Source: CAD feature listing. Evaluate the final solid. Frame: model axes, mm. A direction names the side the tool comes from. Give positions to 0.01 mm unless a question says otherwise; leave off trailing zeros. Order: outer loops, then holes, each group sorted by start corner. A loop starts at its lowest first (then second) coordinate and runs counter-clockwise, first axis right, second up. Notation, with made-up numbers: (-33, -34) - (20, -34) arc R10 cw to (20, -27) - close; hole circle Ø8 at (-37.5, 57.25). An arc over 180 degrees is marked (long way). Write each question's results on one line, items separated by ' | '. Start each with the question number.
Item 1: Line query: line 1 along Y through (x, z) = (242, 18.25); line 2 along X through (y, z) = (0, 18); line 3 along Z through (x, y) = (-39, -187.5). Output: solid intervals per line, ascending.
Item 2: Section B-B on x = -57. Output: boundary loops of the cut face in (y, z), and give its area (3 significant figures).
Item 3: Mould query, pull axis Y, two halves, no side actions, for faces 4 (the cylindrical face through (-57.08, -126.19, 31.67)), 5 (the flat face through (0.88, 133.23, 37.99)), 6 (the flat face through (4, -26, 18.5)), 7 (the cylindrical face through (57.08, 126.19, 31.67)). Classes: released by +Y, released by -Y, zero draft, split by the parting line, or undercut.
Item 4: Section A-A on z = 42.5. Output: boundary loops of the cut face in (x, y).
Item 5: Set-up query: faces 1 (the cylindrical face through (-28.53, -205.21, 57.52)), 2 (the flat face through (1, 180, 57.031)), 3 (the flat face through (1, -179, 57.031)). Return all of +Z, -Z, +X, -X, +Y, -Y with unobstructed straight access to the full face (end or side cutting, diameter ignored); none if empty.
Item 6: Contact query for flat-ended pins moving along their axis: pin 1 Ø3 at (x, y) = (13.5, -41.5) entering from +Z; pin 2 Ø0.5 at (y, z) = (-206.5, 57.5) entering from -X; pin 3 Ø1.1 at (y, z) = (198.5, 57.5) entering from -X. Output: stop coordinate, or through.
Item 7: Section C-C on y = 53.5. Output: boundary loops of the cut face in (x, z), and give its area (3 significant figures).
Item 8: Section D-D on x = 123. Output: boundary loops of the cut face in (y, z).
```python
from build123d import *

# Parameters (mm, degrees)
SALIENTE_EXTRUIR1_DEPTH     = 271
CORTAR_EXTRUIR9_DEPTH       = 372.904084134
CORTAR_EXTRUIR9_DEPTH_BACK  = 372.904084134
CROQUIS4_R                  = 2.5
CORTAR_EXTRUIR10_DEPTH      = 372.904084134
CORTAR_EXTRUIR10_DEPTH_BACK = 372.904084134
CROQUIS2_W                  = 600.899293422
CROQUIS2_H                  = 554.061756016


with BuildPart() as part:
    # Croquis1 → Saliente-Extruir1 (new, symmetric)
    with BuildSketch(Plane(origin=(0, 0, 0), x_dir=(0, 0, -1), z_dir=(1, 0, 0))):
        Polygon((-18.5, -110), (-18.5, 110), (-58.031437996, 157.111733252), (-58.031437996, 248), (-57.031437996, 248), (-57.031437996, 157.475703486), (-17.5, 110.363970234), (-17.5, -110.363970234), (-57.031437996, -157.475703486), (-57.031437996, -248), (-58.031437996, -248), (-58.031437996, -157.111733252), align=None)
    extrude(amount=SALIENTE_EXTRUIR1_DEPTH, both=True)

    # Croquis4 → Cortar-Extruir9 (cut, two sides: drawn at the far end of the back side and taken through both)
    with BuildSketch(Plane.XY.offset(-CORTAR_EXTRUIR9_DEPTH_BACK)):
        with Locations(Location((-242, 0, 0), (0, 0, 90))):
            Circle(CROQUIS4_R)
        with Locations(Location((242, 0, 0), (0, 0, 90))):
            Circle(CROQUIS4_R)
        with BuildLine():
            Line((-5, 201.31662479), (-5, 194.68337521))
            ThreePointArc((-5, 194.68337521), (0, 192), (5, 194.68337521))
            Line((5, 194.68337521), (5, 201.31662479))
            ThreePointArc((5, 201.31662479), (0, 204), (-5, 201.31662479))
        make_face()
        with BuildLine():
            Line((5, -201.31662479), (5, -194.68337521))
            ThreePointArc((5, -194.68337521), (0, -192), (-5, -194.68337521))
            Line((-5, -194.68337521), (-5, -201.31662479))
            ThreePointArc((-5, -201.31662479), (0, -204), (5, -201.31662479))
        make_face()
        with BuildLine():
            Line((-5.933205139, 0.892791565), (-3.129872731, -5.118974183))
            ThreePointArc((-3.129872731, -5.118974183), (2.53570957, -5.437846722), (5.933205139, -0.892791565))
            Line((5.933205139, -0.892791565), (3.129872731, 5.118974183))
            ThreePointArc((3.129872731, 5.118974183), (-2.53570957, 5.437846722), (-5.933205139, 0.892791565))
        make_face()
    extrude(amount=CORTAR_EXTRUIR9_DEPTH + CORTAR_EXTRUIR9_DEPTH_BACK, mode=Mode.SUBTRACT)

    # Croquis2 → Cortar-Extruir10 (cut, two sides: drawn at the far end of the back side and taken through both)
    with BuildSketch(Plane.XY.offset(-CORTAR_EXTRUIR10_DEPTH_BACK)):
        Rectangle(CROQUIS2_W, CROQUIS2_H)
        with BuildLine():
            Line((1.5, 198), (1.5, 213.5))
            ThreePointArc((1.5, 213.5), (28.875083063, 204.989128333), (47.85, 183.5))
            ThreePointArc((47.85, 183.5), (49.675606578, 178.308038097), (50.3, 172.84))
            ThreePointArc((50.3, 172.84), (59.704263449, 118.077622514), (86.695218386, 69.509664861))
            ThreePointArc((86.695218386, 69.509664861), (152.735315328, 25.690942775), (231.948594909, 28.266044217))
            ThreePointArc((231.948594909, 28.266044217), (272, 0), (231.948594909, -28.266044217))
            ThreePointArc((231.948594909, -28.266044217), (152.735315328, -25.690942775), (86.695218386, -69.509664861))
            ThreePointArc((86.695218386, -69.509664861), (59.704263449, -118.077622514), (50.3, -172.84))
            ThreePointArc((50.3, -172.84), (49.675606578, -178.308038097), (47.85, -183.5))
            ThreePointArc((47.85, -183.5), (28.875083063, -204.989128333), (1.5, -213.5))
            Line((1.5, -213.5), (1.5, -198))
            Line((1.5, -198), (-1.5, -198))
            Line((-1.5, -198), (-1.5, -213.5))
            ThreePointArc((-1.5, -213.5), (-28.875083063, -204.989128333), (-47.85, -183.5))
            ThreePointArc((-47.85, -183.5), (-49.675606578, -178.308038097), (-50.3, -172.84))
            ThreePointArc((-50.3, -172.84), (-59.704263449, -118.077622514), (-86.695218386, -69.509664861))
            ThreePointArc((-86.695218386, -69.509664861), (-152.735315328, -25.690942775), (-231.948594909, -28.266044217))
            ThreePointArc((-231.948594909, -28.266044217), (-272, 0), (-231.948594909, 28.266044217))
            ThreePointArc((-231.948594909, 28.266044217), (-152.735315328, 25.690942775), (-86.695218386, 69.509664861))
            ThreePointArc((-86.695218386, 69.509664861), (-59.704263449, 118.077622514), (-50.3, 172.84))
            ThreePointArc((-50.3, 172.84), (-49.675606578, 178.308038097), (-47.85, 183.5))
            ThreePointArc((-47.85, 183.5), (-28.875083063, 204.989128333), (-1.5, 213.5))
            Line((-1.5, 213.5), (-1.5, 198))
            Line((-1.5, 198), (1.5, 198))
        make_face(mode=Mode.SUBTRACT)
    extrude(amount=CORTAR_EXTRUIR10_DEPTH + CORTAR_EXTRUIR10_DEPTH_BACK, mode=Mode.SUBTRACT)


solid = part.part
```
Evaluation:
1) line 1: y = -30 to -2.5, 2.5 to 30 | line 2: x = -271 to -244.5, -239.5 to -5.52, 5.52 to 239.5, 244.5 to 271 | line 3: z = 57.03 to 58.03
2) outline: (-126.46, 31.01) - (-110.36, 17.5) - (110.36, 17.5) - (126.46, 31.01) - (126.46, 32.31) - (110, 18.5) - (-110, 18.5) - (-126.46, 32.31) - close | area: 263 mm^2
3) face 4: released by -Y | face 5: undercut | face 6: undercut | face 7: released by +Y
4) outline: (-53.93, -138.6) arc R165.58 cw to (-53.61, -140.16) - (53.61, -140.16) arc R165.58 cw to (53.93, -138.6) - close; (-53.93, 138.6) - (53.93, 138.6) arc R165.58 cw to (53.61, 140.16) - (-53.61, 140.16) arc R165.58 cw to start
5) face 1: +Z, -Z, -X, -Y | face 2: -Z, +X, -X, +Y | face 3: -Z, +X, -X, -Y
6) pin 1: stops at z = 18.5 | pin 2: stops at x = -26.83 | pin 3: stops at x = -37.58
7) outline: (-101.94, 17.5) - (101.94, 17.5) - (101.94, 18.5) - (-101.94, 18.5) - close | area: 204 mm^2
8) outline: (-38.3, 17.5) - (38.3, 17.5) - (38.3, 18.5) - (-38.3, 18.5) - close
